```python
from build123d import *

# Parameters (mm, degrees)
BOSS_EXTRUDE1_DEPTH = 1.5
BOSS_EXTRUDE3_START = -1
SKETCH5_W           = 7.6
SKETCH5_H           = 0.2
BOSS_EXTRUDE3_DEPTH = 0.5
SKETCH6_W           = 0.5
SKETCH6_H           = 1.2
CUT_EXTRUDE2_DEPTH  = 0.5
FILLET2_R           = 0.1


with BuildPart() as part:
    # Sketch1 → Boss-Extrude1 (new body)
    with BuildSketch(Plane.XY):
        with BuildLine():
            Line((-0.6, 0.7), (-0.6, -0.6))
            Line((-0.6, -0.6), (-0.4, -0.6))
            Line((-0.4, -0.6), (-0.4, 0.6))
            Line((-0.4, 0.6), (0.4, 0.6))
            Line((0.4, 0.6), (0.4, -0.6))
            Line((0.4, -0.6), (0.6, -0.6))
            Line((0.6, -0.6), (0.6, 0.7))
            ThreePointArc((0.6, 0.7), (0.570710678, 0.770710678), (0.5, 0.8))
            Line((0.5, 0.8), (-0.5, 0.8))
            ThreePointArc((-0.5, 0.8), (-0.570710678, 0.770710678), (-0.6, 0.7))
        make_face()
    extrude(amount=BOSS_EXTRUDE1_DEPTH)

    # Sketch5 → Boss-Extrude3 (add)
    with BuildSketch(Plane.XY.offset(1.5).offset(BOSS_EXTRUDE3_START)):
        with Locations((3.8, 0.7)):
            Rectangle(SKETCH5_W, SKETCH5_H)
    extrude(amount=BOSS_EXTRUDE3_DEPTH)

    # Sketch6 → Cut-Extrude2 (cut)
    with BuildSketch(Plane(origin=(0.6, 0, 0), x_dir=(0, 0, -1), z_dir=(1, 0, 0))):
        with Locations((-0.75, 0)):
            Rectangle(SKETCH6_W, SKETCH6_H)
    extrude(amount=-CUT_EXTRUDE2_DEPTH, mode=Mode.SUBTRACT)

    # Fillet2
    fillet2_edges = [part.edges().sort_by_distance(p)[0] for p in [
        (-0.5, -0.6, 0),
        (0.5, -0.6, 0),
        (-0.5, -0.6, 1.5),
        (7.6, 0.7, 1),
        (7.6, 0.7, 0.5),
        (0.5, -0.6, 0.5),
        (0.5, -0.6, 1),
        (0.5, -0.6, 1.5),
    ]]
    fillet(fillet2_edges, radius=FILLET2_R)


solid = part.part
```
Design review of the part built by this model. Coordinates are the model's own, in mm. Coordinates: 2 decimals unless noted, no trailing zeros. Loops run counter-clockwise (first coordinate to the right, second up) from the corner with the lowest first, then second, coordinate; pieces in that order, holes last. Notation, with made-up numbers: (41.5, 14.5) - (88.5, 14.5) arc R21 cw to (88.5, 50.5) - close; hole circle Ø5 at (-11, 81.25). An arc over 180 degrees is marked (long way). Use CSV: the item, a comma, the result in double quotes. Start each with the question number.
1) Consider section A-A on y = -0.15. Write out the cut boundary in (x, z), then the cut area to 3 significant figures.
2) Consider section D-D on z = 0.2. Write out the cut boundary in (x, y).
3) Consider section C-C on x = 5.5. Write out the cut boundary in (y, z).
4) Wall thickness on L1, parallel to X at y = 0.55, z = 0.1; L2, parallel to Z at x = 0.5, y = -0.2; L3, parallel to X at y = 0.7, z = 1.35: over which ranges is each line inside the solid? List them lowest first. Write a range as from..to.
5) The part is to be moulded in two halves that separate along X. For faces 1 (the flat face through (2.7, 0.6, 0.7)), 2 (the flat face through (-0.6, 0, 1)), 3 (the flat face through (2.7, 0.8, 0.7)), say which applies: +X half, -X half, draft (parallel to the pull), parting line (faces both ways), or undercut.
6) Consider section B-B on z = 0.8. Write out the cut boundary in (x, y), then the cut area to 3 significant figures.
Geometry says:
1,outline,"(-0.6, 0) - (-0.4, 0) - (-0.4, 1.5) - (-0.6, 1.5) - close; (0.4, 0) - (0.6, 0) - (0.6, 0.5) - (0.4, 0.5) - close; (0.4, 1) - (0.6, 1) - (0.6, 1.5) - (0.4, 1.5) - close"
1,area,"0.500 mm^2"
2,outline,"(-0.6, -0.6) - (-0.4, -0.6) - (-0.4, 0.6) - (0.4, 0.6) - (0.4, -0.6) - (0.6, -0.6) - (0.6, 0.7) arc R0.1 ccw to (0.5, 0.8) - (-0.5, 0.8) arc R0.1 ccw to (-0.6, 0.7) - close"
3,outline,"(0.6, 0.5) - (0.8, 0.5) - (0.8, 1) - (0.6, 1) - close"
4,L1,"-0.6..-0.4, 0.4..0.6"
4,L2,"0..0.5, 1..1.5"
4,L3,"-0.6..0.6"
5,face 1,"undercut"
5,face 2,"-X half"
5,face 3,"draft"
6,outline,"(-0.6, -0.6) - (-0.4, -0.6) - (-0.4, 0.6) - (7.6, 0.6) - (7.6, 0.8) - (-0.5, 0.8) arc R0.1 ccw to (-0.6, 0.7) - close"
6,area,"1.88 mm^2"
